```python
from build123d import *

# Parameters (mm, degrees)
SKETCH1_W                    = 303.2
SKETCH1_H                    = 358.2
BOSS_EXTRUDE1_DEPTH          = 92
CHAMFER1_SIZE                = 41
SHELL1_T                     = -1.6
F_7_0_7_DIAMETER_HOLE1_D     = 7
F_7_0_7_DIAMETER_HOLE1_DEPTH = 1.6
F_7_0_7_DIAMETER_HOLE2_D     = 7


with BuildPart() as part:
    # Sketch1 → Boss-Extrude1 (new body)
    with BuildSketch(Plane(origin=(0, 0, 0), x_dir=(1, 0, 0), z_dir=(0, 1, 0))):
        with Locations((0, 179.1)):
            Rectangle(SKETCH1_W, SKETCH1_H)
    extrude(amount=BOSS_EXTRUDE1_DEPTH)

    # Chamfer1
    chamfer1_edges = [part.edges().sort_by_distance(p)[0] for p in [
        (-151.6, 46, -358.2),
        (151.6, 46, -358.2),
    ]]
    chamfer(chamfer1_edges, length=CHAMFER1_SIZE)

    # Shell1
    shell1_openings = [part.faces().sort_by_distance(p)[0] for p in [
        (0, 0, -176.499178778),
    ]]
    offset(amount=SHELL1_T, openings=shell1_openings, kind=Kind.INTERSECTION)

    # Ø7.0 (7) Diameter Hole1
    with Locations(Plane.XY):
        with Locations((-125, 6), (0, 6), (125, 6)):
            Hole(F_7_0_7_DIAMETER_HOLE1_D / 2, depth=F_7_0_7_DIAMETER_HOLE1_DEPTH)

    # Ø7.0 (7) Diameter Hole2 (through all)
    with Locations(Plane.ZY.offset(151.6)):
        with Locations((-8.6, 6), (-88.6, 6), (-178.6, 6)):
            Hole(F_7_0_7_DIAMETER_HOLE2_D / 2)


solid = part.part
```
Could you check a few things on this model? Use its own coordinates, in mm. A direction names the side the tool comes from. Give positions to 0.01 mm unless a question says otherwise; leave off trailing zeros. Loops run counter-clockwise (first coordinate to the right, second up) from the corner with the lowest first, then second, coordinate; pieces in that order, holes last. Notation, with made-up numbers: (-17, 9.25) -> (32, 9.25) arc R30 ccw to (32, 47.25) -> close; hole circle Ø5 at (38, -21). An arc over 180 degrees is marked (long way). Put each result on its own line as item: value.
(1) Please list where these lines run through material, in increasing order: probe 1 along X at (y, z) = (15, -217); probe 2 along Z at (x, y) = (-14, 48.5); probe 3 along Y at (x, z) = (125, -0.7). Write a range as [from, to].
Computed:
probe 1: [-151.6, -150], [150, 151.6]
probe 2: [-358.2, -356.6], [-1.6, 0]
probe 3: [0, 2.5], [9.5, 92]
(2) I'm going to push flat-ended pins straight in: pin 1 Ø3 at (x, z) = (16.5, -282.5) entering from -Y; pin 2 Ø4 at (x, y) = (-125, 6) entering from -Z; pin 3 Ø11 at (x, y) = (125, 6) entering from -Z. Where does each tip first touch, or does it pass through?
Computed:
pin 1: y = 90.4
pin 2: z = -345.8
pin 3: z = -349.3
(3) Imagine slicing it at B-B on z = -301. Write out the boundary of the cut face in (x, y).
Computed:
outline: (-151.6, 0) -> (-150, 0) -> (-150, 90.4) -> (150, 90.4) -> (150, 0) -> (151.6, 0) -> (151.6, 92) -> (-151.6, 92) -> close
(4) Imagine slicing it at A-A on y = 18.5. Write out the boundary of the cut face in (x, z).
Computed:
outline: (-151.6, -317.2) -> (-110.6, -358.2) -> (110.6, -358.2) -> (151.6, -317.2) -> (151.6, 0) -> (-151.6, 0) -> close; hole (-150, -316.54) -> (-109.94, -356.6) -> (109.94, -356.6) -> (150, -316.54) -> (150, -1.6) -> (-150, -1.6) -> close
(5) Thinking about a two-plate mould opening in X: for faces 3 (the face through (-151.6, 45, -156)), 4 (the face through (-2, 45, 0)), 5 (the face through (129.69, 44.57, -336.85)), which applies, pulls with the +X half, pulls with the -X half, needs draft (parallel to the pull), parting line crosses it, or undercut?
Computed:
face 3: pulls with the -X half
face 4: needs draft
face 5: undercut
(6) Imagine slicing it at C-C on x = 96. Write out the boundary of the cut face in (y, z), plus the area to 3 significant figures.
Computed:
outline: (0, -358.2) -> (92, -358.2) -> (92, 0) -> (0, 0) -> (0, -1.6) -> (90.4, -1.6) -> (90.4, -356.6) -> (0, -356.6) -> close
area: 862 mm^2
(7) For faces 1 (the face through (-129.69, 44.57, -336.85)), 2 (the face through (-2, 45, -358.2)), which set-ups out of +Z, -Z, +X, -X, +Y, -Y let a thin tool reach every point of the face, with its end or its side?
Computed:
face 1: -Y
face 2: -Z, +X, -X, +Y, -Y
